The model under review builds one solid part; all positions refer to its coordinate system, in mm. Face numbers are marked on the shaded views. Give positions to 0.01 mm unless a question says otherwise; leave off trailing zeros. Order: outer loops, then holes, each group sorted by start corner. A loop starts at its lowest first (then second) coordinate and runs counter-clockwise, first axis right, second up. Notation, with made-up numbers: (73, -29.5) - (130, -29.5) arc R25 ccw to (130, 0.5) - close; hole circle Ø4 at (9, -28.5). An arc over 180 degrees is marked (long way). Use CSV: the item, a comma, the result in double quotes. Start each with the question number.
1. Take a section at A-A, the plane z = 13.5. Count the separate pieces of the cut face and the enclosed holes in it, then the cut area to 3 significant figures.
2. Draft analysis for pull direction X (two halves, no side actions). For the marked faces 1, 2, 3 and 4, state which applies: released by +X, released by -X, zero draft, split by the parting line, or undercut.
3. For pin 1 (1.5 mm diameter, centred on x = -33.5, z = 7.5, fed in from -Y); pin 2 (5 mm diameter, centred on y = 0, z = 16.5, fed in from -X); pin 3 (16 mm diameter, centred on x = 11.5, y = 6.5, fed in from +Z), all flat-tipped, find the tip position at first contact; note any pin that passes through.
4. To check wall thickness, follow line 1 (X direction, y = -6, z = 10.5); line 2 (X direction, y = 0, z = 26); line 3 (Z direction, x = 5, y = 17.5). State the ranges of each line that lie inside material, in increasing order. Write a range as [from, to].
5. Take a section at D-D, the plane z = 38.5. State the section outline as (x, y) points (1 decimal), then the cut area to 3 significant figures.
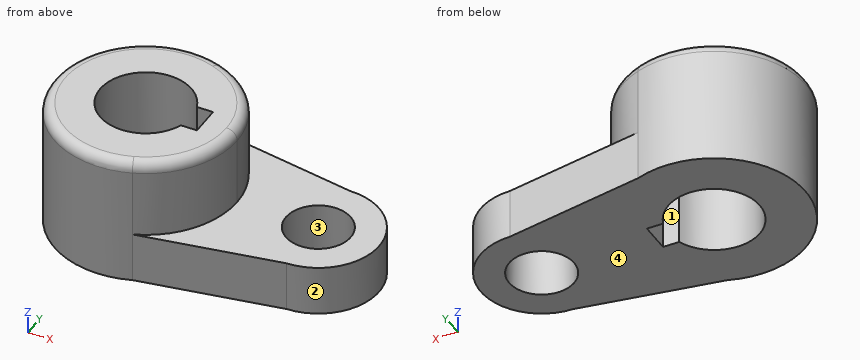
```python
from build123d import *

# Parameters (mm, degrees)
F1_DEPTH = 40.2336
F2_DEPTH = 15.7734
F3_R     = 3.302


with BuildPart() as f1:
    # F0 (on Top) → F1 (new body)
    with BuildSketch(Plane.XY):
        with BuildLine():
            ThreePointArc((-29.8803903858, -26.8489932886), (-16.251542955, -16.3866864902), (-11.0860950838, 0))
            ThreePointArc((-11.0860950838, 0), (-16.251542955, 16.3866864902), (-29.8803903858, 26.8489932886))
            ThreePointArc((-29.8803903858, 26.8489932886), (-68.2360950838, 0), (-29.8803903858, -26.8489932886))
        make_face()
        with BuildLine():
            Line((-21.1405511945, 4.826), (-21.1405511945, 0))
            Line((-21.1405511945, 0), (-21.1405511945, -4.826))
            Line((-21.1405511945, -4.826), (-26.2133302045, -4.826))
            ThreePointArc((-26.2133302045, -4.826), (-53.9485950838, 0), (-26.2133302045, 4.826))
            Line((-26.2133302045, 4.826), (-21.1405511945, 4.826))
        make_face(mode=Mode.SUBTRACT)
    extrude(amount=F1_DEPTH)

    # F0 (on Top) → F2 (join)
    with BuildSketch(Plane.XY):
        with BuildLine():
            ThreePointArc((-29.8803903858, -26.8489932886), (-16.251542955, -16.3866864902), (-11.0860950838, 0))
            ThreePointArc((-11.0860950838, 0), (-16.251542955, 16.3866864902), (-29.8803903858, 26.8489932886))
            ThreePointArc((-29.8803903858, 26.8489932886), (-68.2360950838, 0), (-29.8803903858, -26.8489932886))
        make_face()
        with BuildLine():
            Line((-21.1405511945, 4.826), (-21.1405511945, 0))
            Line((-21.1405511945, 0), (-21.1405511945, -4.826))
            Line((-21.1405511945, -4.826), (-26.2133302045, -4.826))
            ThreePointArc((-26.2133302045, -4.826), (-53.9485950838, 0), (-26.2133302045, 4.826))
            Line((-26.2133302045, 4.826), (-21.1405511945, 4.826))
        make_face(mode=Mode.SUBTRACT)
        with BuildLine():
            ThreePointArc((-29.8803903858, 26.8489932886), (-16.251542955, 16.3866864902), (-11.0860950838, 0))
            ThreePointArc((-11.0860950838, 0), (-16.251542955, -16.3866864902), (-29.8803903858, -26.8489932886))
            Line((-29.8803903858, -26.8489932886), (14.3139049162, -19.05))
            ThreePointArc((14.3139049162, -19.05), (33.3639049162, 0), (14.3139049162, 19.05))
            Line((14.3139049162, 19.05), (-29.8803903858, 26.8489932886))
        make_face()
        with BuildLine():
            ThreePointArc((24.4739049162, 0), (14.3139049162, -10.16), (4.1539049162, 0))
            ThreePointArc((4.1539049162, 0), (14.3139049162, 10.16), (24.4739049162, 0))
        make_face(mode=Mode.SUBTRACT)
    extrude(amount=F2_DEPTH)

    # F3
    f3_edges = [f1.edges().sort_by_distance(p)[0] for p in [
        (-49.4418, 26.848993, 40.2336),
    ]]
    fillet(f3_edges, radius=F3_R)


solid = f1.part
```
Determined:
1,separate pieces,"1"
1,enclosed holes,"2"
1,area,"3,420 mm²"
2,face 1,"undercut"
2,face 2,"released by +X"
2,face 3,"undercut"
2,face 4,"zero draft"
3,pin 1,"stops at y = -28.06"
3,pin 2,"stops at x = -68.24"
3,pin 3,"stops at z = 15.77"
4,line 1,"x = [-67.6, -52.63], [-26.69, 6.11], [22.51, 32.39]"
4,line 2,"x = [-68.24, -53.95], [-21.14, -11.09]"
4,line 3,"z = [0, 15.77]"
5,outline,"circle Ø56.4 at (-39.7, 0); hole (-26.2, -4.8) - (-21.1, -4.8) - (-21.1, 4.8) - (-26.2, 4.8) arc R14.3 ccw (long way) to start"
5,area,"1,810 mm²"
